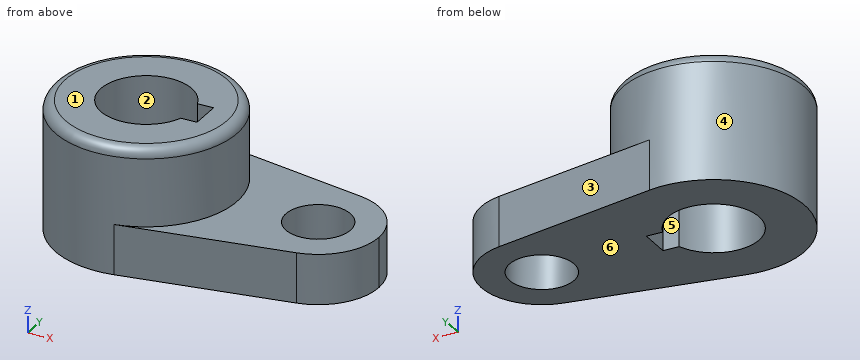
from build123d import *

# Parameters (mm, degrees)
F0_R     = 10.16
F1_DEPTH = 15.76169
F2_DEPTH = 40.2358
F3_R     = 3.175


# Not quite as in the source:
# - a feature names something its author has since deleted; it is built from what else it names


with BuildPart() as f1:
    # F0 (on Top) → F1 (new body)
    with BuildSketch(Plane.XY):
        with BuildLine():
            ThreePointArc((5.0426470588, -28.1265414802), (21.9160245563, -18.3362616868), (28.575, 0))
            ThreePointArc((28.575, 0), (21.9160245563, 18.3362616868), (5.0426470588, 28.1265414802))
            ThreePointArc((5.0426470588, 28.1265414802), (-28.575, 0), (5.0426470588, -28.1265414802))
        make_face()
        with BuildLine():
            ThreePointArc((-13.4477648793, 4.826), (0, 14.2875), (13.4477648793, 4.826))
            Line((13.4477648793, 4.826), (18.5277648793, 4.826))
            Line((18.5277648793, 4.826), (18.5277648793, -4.826))
            Line((18.5277648793, -4.826), (13.4477648793, -4.826))
            ThreePointArc((13.4477648793, -4.826), (0, -14.2875), (-13.4477648793, -4.826))
            Line((-13.4477648793, -4.826), (-18.5277648793, -4.826))
            Line((-18.5277648793, -4.826), (-18.5277648793, 4.826))
            Line((-18.5277648793, 4.826), (-13.4477648793, 4.826))
        make_face(mode=Mode.SUBTRACT)
        with BuildLine():
            ThreePointArc((5.0426470588, 28.1265414802), (21.9160245563, 18.3362616868), (28.575, 0))
            ThreePointArc((28.575, 0), (21.9160245563, -18.3362616868), (5.0426470588, -28.1265414802))
            Line((5.0426470588, -28.1265414802), (57.3367647059, -18.7510276535))
            ThreePointArc((57.3367647059, -18.7510276535), (34.925, 0), (57.3367647059, 18.7510276535))
            Line((57.3367647059, 18.7510276535), (5.0426470588, 28.1265414802))
        make_face()
        with BuildLine():
            ThreePointArc((-13.4477648793, -4.826), (-14.2875, 0), (-13.4477648793, 4.826))
            Line((-13.4477648793, 4.826), (-18.5277648793, 4.826))
            Line((-18.5277648793, 4.826), (-18.5277648793, -4.826))
            Line((-18.5277648793, -4.826), (-13.4477648793, -4.826))
        make_face()
        with BuildLine():
            ThreePointArc((73.025, 0), (68.5856830375, 12.2241744579), (57.3367647059, 18.7510276535))
            ThreePointArc((57.3367647059, 18.7510276535), (34.925, 0), (57.3367647059, -18.7510276535))
            ThreePointArc((57.3367647059, -18.7510276535), (68.5856830375, -12.2241744579), (73.025, 0))
        make_face()
        with Locations((53.975, 0)):
            Circle(F0_R, mode=Mode.SUBTRACT)
    extrude(amount=F1_DEPTH)

    # F0 (on Top) → F2 (join)
    with BuildSketch(Plane.XY):
        with BuildLine():
            ThreePointArc((5.0426470588, -28.1265414802), (21.9160245563, -18.3362616868), (28.575, 0))
            ThreePointArc((28.575, 0), (21.9160245563, 18.3362616868), (5.0426470588, 28.1265414802))
            ThreePointArc((5.0426470588, 28.1265414802), (-28.575, 0), (5.0426470588, -28.1265414802))
        make_face()
        with BuildLine():
            ThreePointArc((-13.4477648793, 4.826), (0, 14.2875), (13.4477648793, 4.826))
            Line((13.4477648793, 4.826), (18.5277648793, 4.826))
            Line((18.5277648793, 4.826), (18.5277648793, -4.826))
            Line((18.5277648793, -4.826), (13.4477648793, -4.826))
            ThreePointArc((13.4477648793, -4.826), (0, -14.2875), (-13.4477648793, -4.826))
            Line((-13.4477648793, -4.826), (-18.5277648793, -4.826))
            Line((-18.5277648793, -4.826), (-18.5277648793, 4.826))
            Line((-18.5277648793, 4.826), (-13.4477648793, 4.826))
        make_face(mode=Mode.SUBTRACT)
        with BuildLine():
            ThreePointArc((-13.4477648793, -4.826), (-14.2875, 0), (-13.4477648793, 4.826))
            Line((-13.4477648793, 4.826), (-18.5277648793, 4.826))
            Line((-18.5277648793, 4.826), (-18.5277648793, -4.826))
            Line((-18.5277648793, -4.826), (-13.4477648793, -4.826))
        make_face()
    extrude(amount=F2_DEPTH)

    # F3
    f3_edges = [f1.edges().sort_by_distance(p)[0] for p in [
        (-5.042647, 28.126541, 40.2358),
    ]]
    fillet(f3_edges, radius=F3_R)


solid = f1.part
The listing builds one solid part. Answer for the finished solid, in the listing's coordinates (mm). Face numbers are marked on the shaded views. A direction names the side the tool comes from. Give positions to 0.01 mm unless a question says otherwise; leave off trailing zeros. Loops run counter-clockwise (first coordinate to the right, second up) from the corner with the lowest first, then second, coordinate; pieces in that order, holes last.
Item 1: A cutting plane is placed at C-C (x = 41). Give the vertices of the cut face in (y, z), then the cut area to 3 significant figures.
Derived:
outline: (-21.68, 0) - (21.68, 0) - (21.68, 15.76) - (-21.68, 15.76) - close
area: 683 mm2
Item 2: Find the intervals of material crossed by line 1 along X through (y, z) = (-0.5, 28); line 2 along Y through (x, z) = (6, 20); line 3 along Y through (x, z) = (50.5, 7.5), in increasing order.
Derived:
line 1: x = -28.57 to -14.28, 18.53 to 28.57
line 2: y = -27.94 to -12.97, 12.97 to 27.94
line 3: y = -19.98 to -9.55, 9.55 to 19.98
Item 3: A tool of negligible diameter and unlimited length cuts with its end or side. For the marked faces 4, 5 and 6, from which of +Z, -Z, +X, -X, +Y, -Y can it reach the whole face along a straight path? Write none if from no direction.
Derived:
face 4: +Z
face 5: +Z, -Z
face 6: -Z, +X, -X, +Y, -Y
Item 4: A cutting plane is placed at B-B (y = 1). Give the number of separate pieces and of enclosed holes in the cut face, then the cut area to 3 significant figures.
Derived:
separate pieces: 3
enclosed holes: 0
area: 1,360 mm2
Item 5: Determine the mould class of the marked faces 1, 2 and 3 for opening direction Y: +Y half, -Y half, draft (parallel to the pull), parting line (faces both ways), or undercut.
Derived:
face 1: draft
face 2: undercut
face 3: +Y half
Item 6: Each of these flat-tipped pins is pushed along its axis until it touches: pin 1 Ø1 at (x, y) = (16, -20.5) entering from +Z; pin 2 Ø3 at (x, y) = (39, 7.5) entering from +Z; pin 3 Ø12 at (y, z) = (-22, 18.5) entering from +X; pin 4 Ø12 at (y, z) = (-22, 15) entering from -X. Where does it stop, or does it pass through?
Derived:
pin 1: stops at z = 40.23
pin 2: stops at z = 15.76
pin 3: stops at x = 63.21
pin 4: stops at x = -23.68
